The model under review builds one solid part; all positions refer to its coordinate system, in mm. Coordinates: 2 decimals unless noted, no trailing zeros. Order: outer loops, then holes, each group sorted by start corner. A loop starts at its lowest first (then second) coordinate and runs counter-clockwise, first axis right, second up. Notation, with made-up numbers: M -5,14 L 36,14 A20 cw 36,41 Z; hole C -35.5,-7 d1. An arc over 180 degrees is marked long. One line per item, written item: value.
```python
from build123d import *

# Parameters (mm, degrees)
SKETCH1_W           = 7.5
SKETCH1_H           = 7.5
SKETCH1_R           = 1.56
BOSS_EXTRUDE1_DEPTH = 7.4
CUT_EXTRUDE1_DEPTH  = 8.5


with BuildPart() as part:
    # Sketch1 → Boss-Extrude1 (new body)
    with BuildSketch(Plane.XY):
        Rectangle(SKETCH1_W, SKETCH1_H)
        Circle(SKETCH1_R, mode=Mode.SUBTRACT)
    extrude(amount=BOSS_EXTRUDE1_DEPTH)

    # Sketch2 → Cut-Extrude1 (cut, through all)
    with BuildSketch(Plane(origin=(3.75, 0, 0), x_dir=(0, 0, -1), z_dir=(1, 0, 0))):
        Polygon((-3.7, 3.12), (-4.33, 3.75), (-3.07, 3.75), align=None)
    extrude(amount=-CUT_EXTRUDE1_DEPTH, mode=Mode.SUBTRACT)


solid = part.part
```
(1) Mouldability with a two-part tool opening along Y and no side actions: class faces 1 (the flat face through (-2, 0, 0)), 2 (the cylindrical face through (1.488, 0.469, 3.648)), 3 (the flat face through (0, 3.75, 6)) as +Y half, -Y half, draft (parallel to the pull), parting line (faces both ways), or undercut.
Geometry results:
face 1: draft
face 2: undercut
face 3: +Y half
(2) For L1, parallel to Y at x = 0, z = 2.25; L2, parallel to Z at x = -1.25, y = 3.25; L3, parallel to X at y = 1.25, z = 3.25, list the stretches that pass through material, from the lowest coordinate up.
Geometry results:
L1: y = -3.75 to -1.56, 1.56 to 3.75
L2: z = 0 to 3.57, 3.83 to 7.4
L3: x = -3.75 to -0.93, 0.93 to 3.75
(3) We need section B-B, the plane x = 0. State the section outline as (y, z) points.
Geometry results:
outline: M -3.75,0 L -1.56,0 L -1.56,7.4 L -3.75,7.4 Z; M 1.56,0 L 3.75,0 L 3.75,3.07 L 3.12,3.7 L 3.75,4.33 L 3.75,7.4 L 1.56,7.4 Z
(4) We need section C-C, the plane z = 2.5. State the section outline as (x, y) points, plus the area to 3 significant figures.
Geometry results:
outline: M -3.75,-3.75 L 3.75,-3.75 L 3.75,3.75 L -3.75,3.75 Z; hole C 0,0 d3.12
area: 48.6 mm2
(5) We need section D-D, the plane y = 0. State the section outline as (x, z) points, plus the area to 3 significant figures.
Geometry results:
outline: M -3.75,0 L -1.56,0 L -1.56,7.4 L -3.75,7.4 Z; M 1.56,0 L 3.75,0 L 3.75,7.4 L 1.56,7.4 Z
area: 32.4 mm2
(6) We need section A-A, the plane y = 3.25. State the section outline as (x, z) points, plus the area to 4 significant figures.
Geometry results:
outline: M -3.75,0 L 3.75,0 L 3.75,3.57 L -3.75,3.57 Z; M -3.75,3.83 L 3.75,3.83 L 3.75,7.4 L -3.75,7.4 Z
area: 53.55 mm2
